```python
from build123d import *

# Parameters (mm, degrees)
EXTRUDE_1_DEPTH     = 6
SKETCH_2_R          = 5.5
EXTRUDE_2_DEPTH     = 12
SKETCH_3_R          = 1.6
CUT_EXTRUDE_1_DEPTH = 6
CUT_EXTRUDE_2_DEPTH = 12
SKETCH_5_R          = 1.5
CUT_EXTRUDE_3_DEPTH = 10
CUT_EXTRUDE_4_DEPTH = 12


with BuildPart() as part:
    # 草图1 → 凸台-拉伸1 (new body)
    with BuildSketch(Plane.XY):
        Polygon((5.429941256, -4.302991745), (6.441470791, 2.550971196), (1.011529536, 6.853962941), (-5.429941256, 4.302991745), (-6.441470791, -2.550971196), (-1.011529536, -6.853962941), align=None)
    extrude(amount=EXTRUDE_1_DEPTH)

    # 草图2 → 凸台-拉伸2 (add)
    with BuildSketch(Plane.XY.offset(6)):
        Circle(SKETCH_2_R)
    extrude(amount=EXTRUDE_2_DEPTH)

    # 草图3 → 切除-拉伸1 (cut)
    with BuildSketch(Plane(origin=(0, 0, 0), x_dir=(-1, 0, 0), z_dir=(0, 0, -1))):
        Circle(SKETCH_3_R)
    extrude(amount=-CUT_EXTRUDE_1_DEPTH, mode=Mode.SUBTRACT)

    # 草图4 → 切除-拉伸2 (cut)
    with BuildSketch(Plane.XY.offset(18)):
        with BuildLine():
            Line((2.45, 1.731328969), (2.45, -1.731328969))
            ThreePointArc((2.45, -1.731328969), (-3, 0), (2.45, 1.731328969))
        make_face()
    extrude(amount=-CUT_EXTRUDE_2_DEPTH, mode=Mode.SUBTRACT)

    # 草图5 → 切除-拉伸3 (cut)
    with BuildSketch(Plane.ZY.offset(-2.45)):
        with Locations(Location((14.888016114, 0, 0), (0, 0, 270))):
            Circle(SKETCH_5_R)
    extrude(amount=-CUT_EXTRUDE_3_DEPTH, mode=Mode.SUBTRACT)

    # 草图6 → 切除-拉伸4 (cut)
    with BuildSketch(Plane.XY.offset(18)):
        with BuildLine():
            Line((2.569146545, 2.226990352), (2.569146545, -2.226990352))
            ThreePointArc((2.569146545, -2.226990352), (-3.4, 0), (2.569146545, 2.226990352))
        make_face()
    extrude(amount=-CUT_EXTRUDE_4_DEPTH, mode=Mode.SUBTRACT)


solid = part.part
```
CAD build for the part. Positions are in the model's coordinates, mm. A direction names the side the tool comes from. Round coordinates to 2 decimals unless told otherwise and drop trailing zeros. Order: outer loops, then holes, each group sorted by start corner. A loop starts at its lowest first (then second) coordinate and runs counter-clockwise, first axis right, second up. Notation, with made-up numbers: (51, 41.25) -> (73, 41.25) arc R32 cw to (73, 80.25) -> close; hole circle Ø10 at (45, 35). An arc over 180 degrees is marked (long way). One line per question, with ' | ' between items.
Q1. Slice it at C-C (z = 5.5). Write the cut outline in (x, y).
Completed:
outline: (-6.44, -2.55) -> (-1.01, -6.85) -> (5.43, -4.3) -> (6.44, 2.55) -> (1.01, 6.85) -> (-5.43, 4.3) -> close; hole circle Ø3.2 at (0, 0)
Q2. Slice it at A-A (y = 0). Write the cut outline in (x, z) (3 decimals), then the cut area to 3 significant figures.
Completed:
outline: (-6.065, 0) -> (-1.6, 0) -> (-1.6, 6) -> (-3.4, 6) -> (-3.4, 18) -> (-5.5, 18) -> (-5.5, 6) -> (-6.065, 6) -> close; (1.6, 0) -> (6.065, 0) -> (6.065, 6) -> (5.5, 6) -> (5.5, 13.388) -> (2.569, 13.388) -> (2.569, 6) -> (1.6, 6) -> close; (2.569, 16.388) -> (5.5, 16.388) -> (5.5, 18) -> (2.569, 18) -> close | area: 105 mm^2
Q3. Probe probe 1 along Z at (x, y) = (4.7, 0); probe 2 along Z at (x, y) = (-1.75, 0.75); probe 3 along Y at (x, z) = (1, 11.5). List the from-to ranges inside material, lowest first.
Completed:
probe 1: z = 0 to 13.39, 16.39 to 18 | probe 2: z = 0 to 6 | probe 3: y = -5.41 to -3.25, 3.25 to 5.41
Q4. Slice it at B-B (x = 0). Write the cut outline in (y, z), then the cut area to 3 significant figures.
Completed:
outline: (-6.45, 0) -> (-1.6, 0) -> (-1.6, 6) -> (-3.4, 6) -> (-3.4, 18) -> (-5.5, 18) -> (-5.5, 6) -> (-6.45, 6) -> close; (1.6, 0) -> (6.45, 0) -> (6.45, 6) -> (5.5, 6) -> (5.5, 18) -> (3.4, 18) -> (3.4, 6) -> (1.6, 6) -> close | area: 109 mm^2
Q5. Slice it at D-D (x = -4). Write the cut outline in (y, z).
Completed:
outline: (-4.49, 0) -> (4.87, 0) -> (4.87, 6) -> (3.77, 6) -> (3.77, 18) -> (-3.77, 18) -> (-3.77, 6) -> (-4.49, 6) -> close
Q6. Which spindle directions (+Z, -Z, +X, -X, +Y, -Y) get a long thin tool onto all of the face, cutting with end or side? Do faces 1 (the flat face through (0, -6, 6)), 2 (the flat face through (-5.93, 0.92, 2.96)), 3 (the cylindrical face through (4.014, -0.692, 13.557)). Say none if no direction does.
Completed:
face 1: +Z | face 2: +Z, -Z, -X, +Y | face 3: +X
Q7. Drop flat-ended pins along their axis: pin 1 (4 mm diameter, centred on y = -5, z = 14, fed in from -X); pin 2 (3.5 mm diameter, centred on x = 0, y = 0, fed in from +Z); pin 3 (4 mm diameter, centred on y = -2.5, z = 8.5, fed in from +X). Give the stop position or say it passes through.
Completed:
pin 1: stops at x = -4.61 | pin 2: stops at z = 6 | pin 3: stops at x = 5.48
Q8. Two-plate mould, pull along Y, no slides. Class faces 4 (the cylindrical face through (1.27, -0.97, 2.96)), 5 (the flat face through (2.16, -5.6, 2.96)), 6 (the flat face through (3.765, 4.672, 2.958)): released by +Y, released by -Y, zero draft, split by the parting line, or undercut.
Completed:
face 4: undercut | face 5: released by -Y | face 6: released by +Y
